```python
from build123d import *

# Parameters (mm, degrees)
SKETCH1_W           = 7
SKETCH1_H           = 7
BOSS_EXTRUDE1_DEPTH = 3
CUT_EXTRUDE1_DEPTH  = 7
CUT_EXTRUDE2_DEPTH  = 11
SKETCH4_R           = 1.8
CUT_EXTRUDE3_DEPTH  = 0.8
CUT_EXTRUDE4_DEPTH  = 0.4


with BuildPart() as part:
    # Sketch1 → Boss-Extrude1 (new body)
    with BuildSketch(Plane(origin=(0, 0, 0), x_dir=(1, 0, 0), z_dir=(0, 1, 0))):
        with Locations((3.5, 3.5)):
            Rectangle(SKETCH1_W, SKETCH1_H)
    extrude(amount=BOSS_EXTRUDE1_DEPTH)

    # Sketch2 → Cut-Extrude1 (cut)
    with BuildSketch(Plane.XY):
        Polygon((0, 0), (0.7, 3), (0, 3), align=None)
        Polygon((7, 0), (6.3, 3), (7, 3), align=None)
    extrude(amount=-CUT_EXTRUDE1_DEPTH, mode=Mode.SUBTRACT)

    # Sketch3 → Cut-Extrude2 (cut)
    with BuildSketch(Plane(origin=(0, 0, 0), x_dir=(0, 0, -1), z_dir=(1, 0, 0))):
        Polygon((0, 0), (0.7, 3), (0, 3), align=None)
        Polygon((7, 3), (6.3, 3), (7, 0), align=None)
    extrude(amount=CUT_EXTRUDE2_DEPTH, mode=Mode.SUBTRACT)

    # Sketch4 → Cut-Extrude3 (cut)
    with BuildSketch(Plane.XZ):
        with Locations(Location((3.5, -3.5, 0), (0, 0, 270))):
            Circle(SKETCH4_R)
    extrude(amount=-CUT_EXTRUDE3_DEPTH, mode=Mode.SUBTRACT)

    # Sketch5 → Cut-Extrude4 (cut)
    with BuildSketch(Plane(origin=(0, 3, 0), x_dir=(1, 0, 0), z_dir=(0, 1, 0))):
        with BuildLine():
            Line((3.560577146, 3.114540144), (3.560577146, 3.697873477))
            Line((3.560577146, 3.697873477), (5.086218172, 3.697873477))
            Line((5.086218172, 3.697873477), (5.086218172, 2.291423157))
            add(Edge.make_bspline(
                [(5.086218172, 2.291423157), (5.067017117, 2.274133072), (5.027766277, 2.238788642), (4.963724103, 2.188944154), (4.893219701, 2.141357686), (4.816679286, 2.095065493), (4.733944457, 2.050440158), (4.645345204, 2.006860163), (4.550718059, 1.964751709), (4.416901441, 1.91200226), (4.244652022, 1.854606501), (4.034073664, 1.804699023), (3.821829494, 1.774088797), (3.679866665, 1.770285893), (3.60895455, 1.768386298)],
                knots=[0, 0, 0, 0, 0.581799769, 1.189316438, 1.825828404, 2.496525428, 3.203088405, 3.942228803, 4.719818701, 5.534979611, 7.181138583, 8.803804008, 10.403462225, 12, 12, 12, 12], degree=3))
            add(Edge.make_bspline(
                [(3.60895455, 1.768386298), (3.564530426, 1.769053863), (3.476957263, 1.770369833), (3.347679322, 1.780962016), (3.222873793, 1.79908519), (3.10243897, 1.824748474), (2.985967191, 1.855684985), (2.87394395, 1.895149291), (2.766766964, 1.94252304), (2.663465207, 1.995311299), (2.565964473, 2.055942911), (2.474170574, 2.122268485), (2.388747899, 2.194864928), (2.310002684, 2.273878576), (2.236880415, 2.358765244), (2.170234263, 2.449929726), (2.110467262, 2.547477268), (2.056841671, 2.650184243), (2.009134136, 2.757147371), (1.968877334, 2.867524799), (1.933584129, 2.979713967), (1.904576972, 3.094108746), (1.883272633, 3.211081052), (1.866711077, 3.330089662), (1.857815915, 3.451878149), (1.85624329, 3.533798405), (1.855448941, 3.575177163)],
                knots=[0, 0, 0, 0, 1.124918047, 2.217548049, 3.282233239, 4.316494221, 5.334437038, 6.332151046, 7.320712088, 8.300141923, 9.267552434, 10.225301062, 11.165776911, 12.103230934, 13.047553934, 14.000517593, 14.959782875, 15.941944936, 16.932894943, 17.923491392, 18.915624898, 19.910402922, 20.909870877, 21.92519501, 22.95199481, 24, 24, 24, 24], degree=3))
            add(Edge.make_bspline(
                [(1.855448941, 3.575177163), (1.856093148, 3.619838006), (1.857363158, 3.70788383), (1.868308868, 3.838014535), (1.885306261, 3.964331927), (1.911081696, 4.086606684), (1.942440107, 4.205407986), (1.980711267, 4.320657597), (2.027601885, 4.431501631), (2.079763432, 4.538888047), (2.139142377, 4.641331803), (2.206237244, 4.73751889), (2.279062516, 4.828419459), (2.359057277, 4.912589631), (2.445939825, 4.989988393), (2.538826953, 5.06147172), (2.637496219, 5.128271897), (2.70811648, 5.165936981), (2.743770255, 5.184952804)],
                knots=[0, 0, 0, 0, 1.105010302, 2.178452875, 3.229459892, 4.257086284, 5.268538906, 6.268935615, 7.259234261, 8.24469117, 9.221745683, 10.185929258, 11.144249683, 12.101504986, 13.055838221, 14.020611351, 15.000673771, 16, 16, 16, 16], degree=3))
            add(Edge.make_bspline(
                [(2.743770255, 5.184952804), (2.772065201, 5.199002298), (2.829534559, 5.227537973), (2.920968547, 5.261607564), (3.016595835, 5.292607583), (3.117860188, 5.315737399), (3.224073939, 5.33474033), (3.335190018, 5.348921508), (3.4515659, 5.356368591), (3.530653011, 5.357533973), (3.571093973, 5.358129887)],
                knots=[0, 0, 0, 0, 0.887969848, 1.803539625, 2.741143579, 3.713741423, 4.722068772, 5.775476617, 6.8624965, 8, 8, 8, 8], degree=3))
            add(Edge.make_bspline(
                [(3.571093973, 5.358129887), (3.623235223, 5.357353239), (3.724640313, 5.3558428), (3.872481342, 5.343256962), (4.011619071, 5.321565683), (4.142247257, 5.29169089), (4.264084488, 5.253279835), (4.376921023, 5.206058081), (4.481449427, 5.150975954), (4.576155731, 5.085825914), (4.662964716, 5.013990372), (4.741649855, 4.935381948), (4.81224282, 4.849884207), (4.874790314, 4.75792735), (4.928800044, 4.659131282), (4.975238097, 4.554397044), (5.013462237, 4.442929528), (5.031935116, 4.365517314), (5.041346377, 4.326078605)],
                knots=[0, 0, 0, 0, 1.271135529, 2.472123572, 3.614091059, 4.701890498, 5.736279567, 6.724681829, 7.680621489, 8.611506429, 9.52200816, 10.424540711, 11.318996785, 12.221421405, 13.131851814, 14.060431888, 15.011860567, 16, 16, 16, 16], degree=3))
            Line((5.041346377, 4.326078605), (4.368269454, 4.191463221))
            add(Edge.make_bspline(
                [(4.368269454, 4.191463221), (4.361604715, 4.213549965), (4.348455309, 4.257126698), (4.322964325, 4.319678226), (4.293604309, 4.3784808), (4.260304833, 4.433960038), (4.222730432, 4.485774386), (4.179973312, 4.533364921), (4.134723148, 4.57890244), (4.084024684, 4.619217322), (4.029984173, 4.655561005), (3.973210536, 4.688333605), (3.91242093, 4.71491127), (3.848466862, 4.736295893), (3.781660913, 4.75445708), (3.71113124, 4.76562628), (3.637669879, 4.774050015), (3.58747979, 4.774545043), (3.56197939, 4.774796554)],
                knots=[0, 0, 0, 0, 1.027736275, 2.027704492, 3.005900071, 3.954421694, 4.908588141, 5.853155543, 6.803277083, 7.766271258, 8.734041521, 9.704274878, 10.683578894, 11.68490234, 12.708089448, 13.76461009, 14.864251086, 16, 16, 16, 16], degree=3))
            add(Edge.make_bspline(
                [(3.56197939, 4.774796554), (3.523383641, 4.773766807), (3.448060748, 4.771757168), (3.338099362, 4.758643838), (3.234360883, 4.735314023), (3.13657404, 4.70313499), (3.044559561, 4.661830949), (2.959560848, 4.609861345), (2.879461483, 4.550301297), (2.806540814, 4.480398046), (2.740410053, 4.402016529), (2.68316205, 4.31422182), (2.635503332, 4.217297709), (2.596468126, 4.11173088), (2.565387773, 3.997516933), (2.544303255, 3.874251546), (2.530527014, 3.742123824), (2.529206604, 3.650935474), (2.528525864, 3.603923157)],
                knots=[0, 0, 0, 0, 1.043810997, 2.037086103, 2.989314757, 3.91471467, 4.817033861, 5.710208705, 6.603920097, 7.511448416, 8.435617211, 9.371747005, 10.338444094, 11.350425613, 12.411431869, 13.5347293, 14.729025275, 16, 16, 16, 16], degree=3))
            add(Edge.make_bspline(
                [(2.528525864, 3.603923157), (2.529235737, 3.553411684), (2.530615417, 3.455239689), (2.544030551, 3.312994813), (2.566098564, 3.1804679), (2.597751337, 3.057826113), (2.637580383, 2.944634337), (2.685456676, 2.840530978), (2.744541809, 2.747447788), (2.811096159, 2.66351894), (2.885483615, 2.590182439), (2.965618207, 2.526245677), (3.051053791, 2.472061589), (3.142578213, 2.428485457), (3.239037142, 2.393797733), (3.341317359, 2.36947923), (3.449114318, 2.354373472), (3.522899335, 2.352616709), (3.560577146, 2.351719631)],
                knots=[0, 0, 0, 0, 1.318042826, 2.561693173, 3.724929596, 4.821196409, 5.862977565, 6.853497791, 7.804600806, 8.73339865, 9.643480846, 10.524649628, 11.404635349, 12.277659519, 13.165160235, 14.075017549, 15.017020959, 16, 16, 16, 16], degree=3))
            add(Edge.make_bspline(
                [(3.560577146, 2.351719631), (3.598739169, 2.352780416), (3.675428288, 2.354912133), (3.790294349, 2.372976278), (3.905609834, 2.399558249), (4.018668414, 2.439657646), (4.128467307, 2.485651373), (4.2309763, 2.53865833), (4.326972813, 2.593911136), (4.384773897, 2.636975114), (4.413141249, 2.658109855)],
                knots=[0, 0, 0, 0, 0.993821502, 1.997150276, 3.023717651, 4.073291794, 5.118404464, 6.123376694, 7.078999408, 8, 8, 8, 8], degree=3))
            Line((4.413141249, 2.658109855), (4.413141249, 3.114540144))
            Line((4.413141249, 3.114540144), (3.560577146, 3.114540144))
        make_face()
    extrude(amount=-CUT_EXTRUDE4_DEPTH, mode=Mode.SUBTRACT)


solid = part.part
```
Input: part model. Units: mm. Frame: model coordinates. A direction names the side the tool comes from. Give positions to 0.01 mm unless a question says otherwise; leave off trailing zeros. Order: outer loops, then holes, each group sorted by start corner. A loop starts at its lowest first (then second) coordinate and runs counter-clockwise, first axis right, second up. Notation, with made-up numbers: M 55,-21.75 L 98,-21.75 A25 ccw 98,16.25 Z; hole C 74,42 d11. An arc over 180 degrees is marked long. One line per question, with ' | ' between items. Start each with the question number.
1. Section query B-B (y = 2.5). Return the cut outline in (x, z).
2. Section query A-A (y = 0.7). Return the cut outline in (x, z), and give its area (3 significant figures).
3. Pull-direction query (X, two-part tool) for faces 3 (the face through (4.6, 2.6, -3.2)), 4 (the face through (0.345, 1.479, -3.451)), 5 (the face through (6.655, 1.479, -3.451)), 6 (the face through (4, 0.8, -3)); classes: released by +X, released by -X, zero draft, split by the parting line, or undercut.
4. Material intervals for probe 1 along Y at (x, z) = (4.5, -3.5); probe 2 along X at (y, z) = (0.3, -3.5); probe 3 along X at (y, z) = (0.4, -4.5), sorted ascending. Write a range as [from, to].
5. First-contact query: pin 1 Ø2 at (x, z) = (3.5, -3.5) entering from -Y. Flat tip, straight axial feed; report the tip coordinate or a pass-through.
6. Access query for faces 1 (the face through (2, 0, -5)), 2 (the face through (4.041, 0.394, -5.217)). Directions: +Z, -Z, +X, -X, +Y, -Y. A direction counts if a zero-diameter tool reaches every point of the face in a straight line with its end or side. Return the directions, or none.
Here are the results:
1) outline: M 0.58,-6.42 L 6.42,-6.42 L 6.42,-0.58 L 0.58,-0.58 Z
2) outline: M 0.16,-6.84 L 6.84,-6.84 L 6.84,-0.16 L 0.16,-0.16 Z; hole C 3.5,-3.5 d3.6 | area: 34.4 mm²
3) face 3: undercut | face 4: released by -X | face 5: released by +X | face 6: undercut
4) probe 1: [0.8, 2.6] | probe 2: [0.07, 1.7], [5.3, 6.93] | probe 3: [0.09, 2], [5, 6.91]
5) pin 1: y = 0.8
6) face 1: +Z, -Z, +X, -X, -Y | face 2: -Y
